```python
from build123d import *

# Parameters (mm, degrees)
SKETCH1_R           = 20.799200533
SKETCH1_R_2         = 14
BOSS_EXTRUDE2_DEPTH = 10
SKETCH1_5_R         = 11
SKETCH1_5_R_2       = 20.799200533
SKETCH1_5_R_3       = 7.5
SKETCH1_5_R_4       = 7
BOSS_EXTRUDE3_DEPTH = 5
FILLET1_R           = 5


with BuildPart() as part:
    # Sketch1 → Boss-Extrude2 (new, symmetric)
    with BuildSketch(Plane.XY):
        Circle(SKETCH1_R)
        Circle(SKETCH1_R_2, mode=Mode.SUBTRACT)
    extrude(amount=BOSS_EXTRUDE2_DEPTH, both=True)

    # Sketch1<5> → Boss-Extrude3 (add, symmetric)
    with BuildSketch(Plane.XY):
        with BuildLine():
            Line((67.531815598, 14.697886629), (68, 19))
            ThreePointArc((68, 19), (63.946467856, 31.071046472), (53.428983707, 38.249055455))
            ThreePointArc((53.428983707, 38.249055455), (28.173712308, 57.097365678), (22, 88))
            Line((22, 88), (12, 88))
            ThreePointArc((12, 88), (0, 100), (-12, 88))
            Line((-12, 88), (-22, 88))
            ThreePointArc((-22, 88), (-28.472570597, 56.960167242), (-54.130188439, 38.330834606))
            ThreePointArc((-54.130188439, 38.330834606), (-68.797617118, 16.161980188), (-48.492972379, -0.993572042))
            ThreePointArc((-48.492972379, -0.993572042), (-39.014510451, -3.809523143), (-33.001122743, -11.658726248))
            ThreePointArc((-33.001122743, -11.658726248), (-28.18429152, -20.752004999), (-20.931196761, -28.051470588))
            ThreePointArc((-20.931196761, -28.051470588), (-14.77228566, -37.934411824), (-16.94430214, -49.375))
            ThreePointArc((-16.94430214, -49.375), (-15.922624494, -72.102480293), (5.70222012, -79.169890081))
            Line((5.70222012, -79.169890081), (45.161092518, -67.432567897))
            ThreePointArc((45.161092518, -67.432567897), (56.523753546, -59.49875448), (60.888650386, -46.345688809))
            Line((60.888650386, -46.345688809), (67.531815598, 14.697886629))
        make_face()
        with Locations((0, -60)):
            Circle(SKETCH1_5_R, mode=Mode.SUBTRACT)
        Circle(SKETCH1_5_R_2, mode=Mode.SUBTRACT)
        with BuildLine():
            ThreePointArc((37.105394377, 20.519068244), (49.519068244, 29.894605623), (58.894605623, 17.480931756))
            Line((58.894605623, 17.480931756), (49.783256009, -47.864757052))
            ThreePointArc((49.783256009, -47.864757052), (37.369582142, -57.240294431), (27.994044763, -44.826620565))
            Line((27.994044763, -44.826620565), (37.105394377, 20.519068244))
        make_face(mode=Mode.SUBTRACT)
        with Locations((-49, 19)):
            Circle(SKETCH1_5_R_3, mode=Mode.SUBTRACT)
        with Locations((0, 88)):
            Circle(SKETCH1_5_R_4, mode=Mode.SUBTRACT)
    extrude(amount=BOSS_EXTRUDE3_DEPTH, both=True)

    # Fillet1
    fillet1_edges = [part.edges().sort_by_distance(p)[0] for p in [
        (-20.799200533, 0, 5),
    ]]
    fillet(fillet1_edges, radius=FILLET1_R - 0.0001)  # a hair under: the kernel refuses the full size


solid = part.part
```
Here's how the part is built. I have some questions about the finished solid (model axes, mm). A direction names the side the tool comes from. Give positions to 0.01 mm unless a question says otherwise; leave off trailing zeros. Write each loop counter-clockwise with the first axis right and the second up, starting at its lowest first coordinate (ties: lowest second). Pieces come first, ordered by that corner, then holes. Notation, with made-up numbers: (50, -13.75) -> (80, -13.75) arc R30 cw to (80, 19.25) -> close; hole circle Ø7 at (57.5, -6.5). An arc over 180 degrees is marked (long way). Write each question's results on one line, items separated by ' | '.
Item 1: Suppose I cut it at D-D on y = 62.5. Write out the boundary of the cut face in (x, z), plus the area to 3 significant figures.
Output:
outline: (-25.43, -5) -> (25.27, -5) -> (25.27, 5) -> (-25.43, 5) -> close | area: 507 mm^2
Item 2: Suppose I cut it at B-B on x = -51. Write out the boundary of the cut face in (y, z), plus the area to 3 significant figures.
Output:
outline: (-0.9, -5) -> (11.77, -5) -> (11.77, 5) -> (-0.9, 5) -> close; (26.23, -5) -> (39.29, -5) -> (39.29, 5) -> (26.23, 5) -> close | area: 257 mm^2
Item 3: For pin 1 Ø8 at (x, z) = (49.5, -7) entering from +Y; pin 2 Ø2 at (x, z) = (-12, 8) entering from -Y; pin 3 Ø10 at (x, z) = (39.5, 4) entering from +Y; pin 4 Ø6 at (x, z) = (0, 7.5) entering from +Y, each with a flat end and sliding along its axis, tell me the tip position at first contact or that it passes through.
Output:
pin 1: stops at y = 41.07 | pin 2: stops at y = -18.41 | pin 3: stops at y = 49.25 | pin 4: stops at y = 100
Item 4: Suppose I cut it at C-C on z = -2.75. Write out the boundary of the cut face in (x, y) (3 decimals).
Output:
outline: (-54.13, 38.331) arc R20 ccw to (-48.493, -0.994) arc R16 cw to (-33.001, -11.659) arc R35 ccw to (-20.931, -28.051) arc R16 cw to (-16.944, -49.375) arc R20 ccw to (5.702, -79.17) -> (45.161, -67.433) arc R22 ccw to (60.889, -46.346) -> (68, 19) arc R20 ccw to (53.429, 38.249) arc R44 cw to (22, 88) -> (12, 88) arc R12 ccw to (-12, 88) -> (-22, 88) arc R44 cw to start; hole circle Ø15 at (-49, 19); hole circle Ø28 at (0, 0); hole circle Ø22 at (0, -60); hole circle Ø14 at (0, 88); hole (27.994, -44.827) arc R11 ccw to (49.783, -47.865) -> (58.895, 17.481) arc R11 ccw to (37.105, 20.519) -> close
Item 5: On a 3-axis mill with a long thin cutter (end or side, diameter ignored), from which of +Z, -Z, +X, -X, +Y, -Y can I reach the whole of each face in a straight line? I mean faces 4 (the face through (-4.509, -20.305, -7.465)), 5 (the face through (37.61, -57.27, 0.07)), 6 (the face through (25.16, -73.38, 0.07)). Say none if no direction works.
Output:
face 4: -Z | face 5: +Z, -Z | face 6: +Z, -Z, +X, -Y
Item 6: Suppose I cut it at A-A on y = -60. Write out the boundary of the cut face in (x, z).
Output:
outline: (-20, -5) -> (-11, -5) -> (-11, 5) -> (-20, 5) -> close; (11, -5) -> (56.14, -5) -> (56.14, 5) -> (11, 5) -> close
Item 7: If I drill on L1, parallel to Y at x = 0, z = -1.75; L2, parallel to X at y = -10, z = -2.5; L3, parallel to Y at x = 1.5, z = 2.75, over which ranges is the centre line in solid material (lowest first)?
Output:
L1: y = -80 to -71, -49 to -14, 14 to 81, 95 to 100 | L2: x = -33.69 to -9.8, 9.8 to 32.85, 55.06 to 64.84 | L3: y = -79.94 to -70.9, -49.1 to -13.92, 13.92 to 81.16, 94.84 to 99.91
Item 8: We'd pull the mould along Y, two halves only. Please class faces 1 (the face through (14, -4, 10)), 2 (the face through (49.279, 29.925, 0.07)), 3 (the face through (17, 88, 0)): pulls with the +Y half, pulls with the -Y half, needs draft (parallel to the pull), parting line crosses it, or undercut.
Output:
face 1: needs draft | face 2: undercut | face 3: pulls with the +Y half
